Could you check a few things on this drawing? It's one solid part, dimensions in mm from its lowest x, y, z. A direction names the side the tool comes from. Coordinates: 2 decimals unless noted, no trailing zeros. Loops run counter-clockwise (first coordinate to the right, second up) from the corner with the lowest first, then second, coordinate; pieces in that order, holes last. Notation, with made-up numbers: M 16,60 L 63,60 A23 ccw 63,79 Z; hole C -30,80 d9. An arc over 180 degrees is marked long. Answer as a JSON object with one key per item and string values. Group by question number.
Item 1: If I drill on line 1 (Y direction, x = 81.5, z = 3) (1 decimal); line 2 (Z direction, x = 95, y = 44.5); line 3 (X direction, y = 28.5, z = 22), over which ranges is the centre line in solid material (lowest first)?
Item 2: We'd pull the mould along Y, two halves only. Please class the marked faces 4, 5 and 6: +Y half, -Y half, draft (parallel to the pull), parting line (faces both ways), or undercut.
Item 3: I'm going to push flat-ended pins straight in: pin 1 Ø20.5 at (x, y) = (9, 29) entering from +Z; pin 2 Ø1.5 at (x, z) = (96, 14) entering from +Y; pin 3 Ø12.5 at (y, z) = (33.5, 5) entering from +X; pin 4 Ø20.5 at (y, z) = (18.5, 33) entering from +X. Where does each tip first touch, or does it pass through?
Item 4: Suppose I cut it at A-A (z = 41.5). Write out the boundary of the cut face in (x, y) (1 decimal).
Item 5: Suppose I cut it at D-D (y = 29). Write out the boundary of the cut face in (x, z).
Item 6: Which directions (+Z, -Z, +X, -X, +Y, -Y) give clear straight access to the entire face, cutting with the end or side of a thin tool? Please do the marked faces 1, 2 and 3.
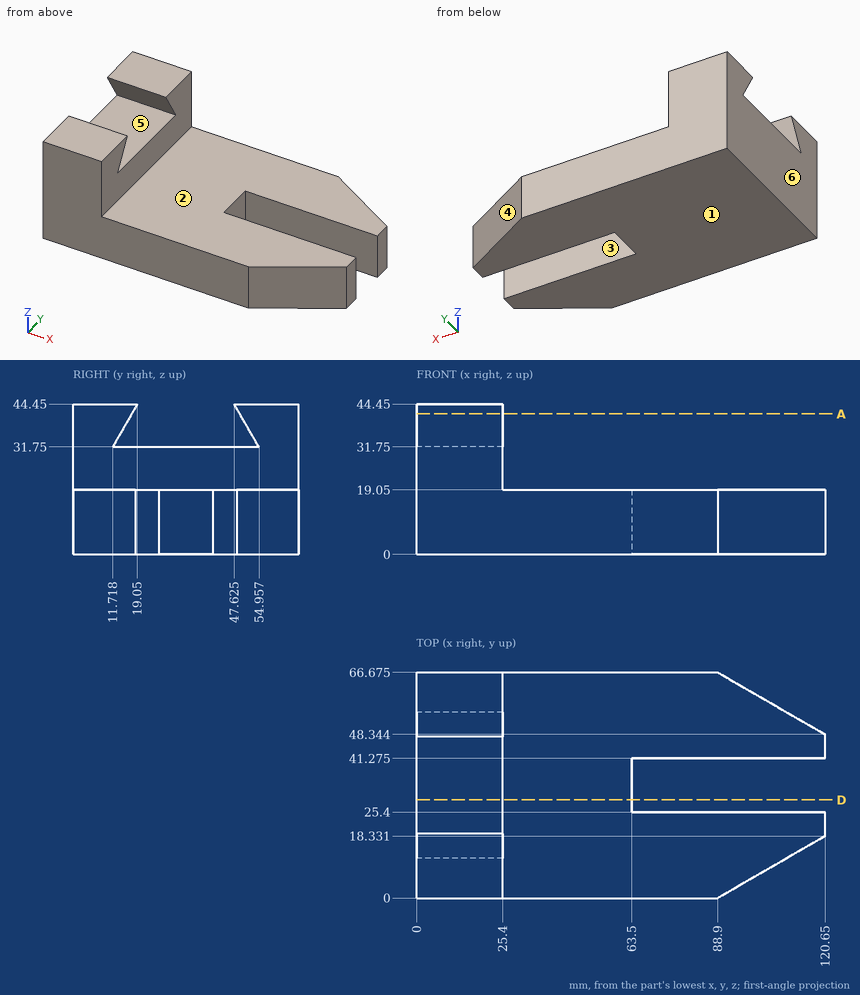
From the geometry:
{
 "1": {"line 1": "0 to 25.4, 41.3 to 66.7", "line 2": "0 to 19.05", "line 3": "0 to 25.4"},
 "2": {"face 4": "+Y half", "face 5": "undercut", "face 6": "draft"},
 "3": {"pin 1": "z = 44.45", "pin 2": "y = 63.01", "pin 3": "x = 63.5", "pin 4": "x = 25.4"},
 "4": {"outline": "M 0,0 L 25.4,0 L 25.4,17.3 L 0,17.3 Z; M 0,49.3 L 25.4,49.3 L 25.4,66.7 L 0,66.7 Z"},
 "5": {"outline": "M 0,0 L 63.5,0 L 63.5,19.05 L 25.4,19.05 L 25.4,31.75 L 0,31.75 Z"},
 "6": {"face 1": "-Z, +X, -X, +Y, -Y", "face 2": "+Z, +X, +Y, -Y", "face 3": "+Z, -Z, +X"}
}
